Check sheet for the modelled part. Datum: model origin and axes. Units: mm. Face numbers are marked on the shaded views. A direction names the side the tool comes from. Give positions to 0.01 mm unless a question says otherwise; leave off trailing zeros. Write each loop counter-clockwise with the first axis right and the second up, starting at its lowest first coordinate (ties: lowest second). Pieces come first, ordered by that corner, then holes. Notation, with made-up numbers: M 1.5,25 L 16.5,25 A13 ccw 16.5,32 Z; hole C -27,85 d1. An arc over 180 degrees is marked long. Write each question's results on one line, items separated by ' | '. Start each with the question number.
from build123d import *

# Parameters (mm, degrees)
SKETCH1_W           = 10
SKETCH1_H           = 10
BOSS_EXTRUDE1_DEPTH = 50
SKETCH3_W           = 10
SKETCH3_H           = 10
BOSS_EXTRUDE3_DEPTH = 11
SKETCH8_W           = 20
SKETCH8_H           = 10
BOSS_EXTRUDE4_DEPTH = 23
SKETCH9_R           = 2
CUT_EXTRUDE2_DEPTH  = 23
SKETCH9_4_R         = 2
CUT_EXTRUDE3_DEPTH  = 23
SKETCH8_4_W         = 20
SKETCH8_4_H         = 10
BOSS_EXTRUDE5_DEPTH = 31
SKETCH8_5_W         = 20
SKETCH8_5_H         = 10
BOSS_EXTRUDE6_DEPTH = 31.5


with BuildPart() as part:
    # Sketch1 → Boss-Extrude1 (new body)
    with BuildSketch(Plane.XY):
        with Locations((-2.851282988, -1.356707317)):
            Rectangle(SKETCH1_W, SKETCH1_H)
    extrude(amount=BOSS_EXTRUDE1_DEPTH)

    # Sketch3 → Boss-Extrude3 (add)
    with BuildSketch(Plane.ZY.offset(7.851282988)):
        with Locations((45, -1.356707317)):
            Rectangle(SKETCH3_W, SKETCH3_H)
    extrude(amount=BOSS_EXTRUDE3_DEPTH)

    # Sketch8 → Boss-Extrude4 (add)
    with BuildSketch(Plane(origin=(0, 3.643292683, 0), x_dir=(1, 0, 0), z_dir=(0, 1, 0))):
        with Locations((-8.851282988, -45)):
            Rectangle(SKETCH8_W, SKETCH8_H)
    extrude(amount=BOSS_EXTRUDE4_DEPTH)

    # Sketch9 → Cut-Extrude2 (cut)
    with BuildSketch(Plane(origin=(0, 3.643292683, 0), x_dir=(1, 0, 0), z_dir=(0, 1, 0))):
        with Locations(Location((-2.851282988, -7, 0), (0, 0, 270))):
            Circle(SKETCH9_R)
    extrude(amount=-CUT_EXTRUDE2_DEPTH, mode=Mode.SUBTRACT)

    # Sketch9<4> → Cut-Extrude3 (cut)
    with BuildSketch(Plane(origin=(0, 3.643292683, 0), x_dir=(1, 0, 0), z_dir=(0, 1, 0))):
        with Locations(Location((-2.851282988, -26, 0), (0, 0, 270))):
            Circle(SKETCH9_4_R)
    extrude(amount=-CUT_EXTRUDE3_DEPTH, mode=Mode.SUBTRACT)

    # Sketch8<4> → Boss-Extrude5 (add)
    with BuildSketch(Plane(origin=(0, 3.643292683, 0), x_dir=(1, 0, 0), z_dir=(0, 1, 0))):
        with Locations((-8.851282988, -45)):
            Rectangle(SKETCH8_4_W, SKETCH8_4_H)
    extrude(amount=BOSS_EXTRUDE5_DEPTH)

    # Sketch8<5> → Boss-Extrude6 (add)
    with BuildSketch(Plane(origin=(0, 3.643292683, 0), x_dir=(1, 0, 0), z_dir=(0, 1, 0))):
        with Locations((-8.851282988, -45)):
            Rectangle(SKETCH8_5_W, SKETCH8_5_H)
    extrude(amount=BOSS_EXTRUDE6_DEPTH)


solid = part.part
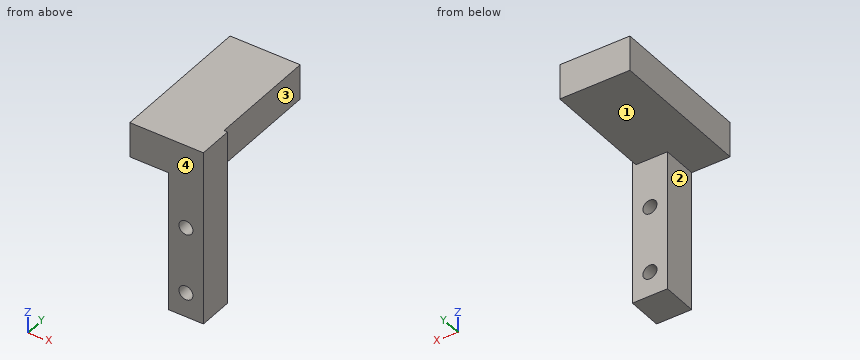
Q1. Tool access check on the marked faces 1, 2, 3 and 4. Record the directions out of +Z, -Z, +X, -X, +Y, -Y that give a thin tool (end or side, any length) a straight path to the whole face; none if there is none.
Q2. Section check B-B on x = -7. Record the boundary of the cut face in (y, z).
Q3. Section check C-C on z = 46. Record the boundary of the cut face in (x, y), plus the area to 3 significant figures.
Q4. Scan lines: L1, parallel to Z at x = -4, y = -4; L2, parallel to X at y = 0.25, z = 7; L3, parallel to Y at x = -4, z = 39.5. Record each from-to range of solid material in increasing order.
Q5. Section check A-A on z = 7. Record the boundary of the cut face in (x, y).
Q6. Section check D-D on y = 29.5. Record the boundary of the cut face in (x, z), plus the area to 3 significant figures.
Q7. Depth check by flat-ended pin: pin 1 Ø6.5 at (x, z) = (-2.85, 7) entering from -Y; pin 2 Ø6.5 at (x, z) = (-2.85, 26) entering from +Y; pin 3 Ø5 at (y, z) = (-1.5, 14) entering from -X; pin 4 Ø5 at (y, z) = (13, 42.5) entering from +X. Enter the tip coordinate at first touch or a pass-through.
Check result:
1) face 1: -Z, -X, +Y | face 2: -Z, -X, +Y, -Y | face 3: +Z, -Z, +X, +Y | face 4: +Z, -Z, +X, -X, -Y
2) outline: M -6.36,0 L 3.64,0 L 3.64,40 L 35.14,40 L 35.14,50 L -6.36,50 Z
3) outline: M -18.85,-6.36 L 2.15,-6.36 L 2.15,3.64 L 1.15,3.64 L 1.15,35.14 L -18.85,35.14 Z | area: 840 mm^2
4) L1: 0 to 5.36, 8.64 to 24.36, 27.64 to 50 | L2: -7.85 to -4.85, -0.85 to 2.15 | L3: -6.36 to 3.64
5) outline: M -7.85,-6.36 L -4.85,-6.36 L -4.85,3.64 L -7.85,3.64 Z; M -0.85,-6.36 L 2.15,-6.36 L 2.15,3.64 L -0.85,3.64 Z
6) outline: M -18.85,40 L 1.15,40 L 1.15,50 L -18.85,50 Z | area: 200 mm^2
7) pin 1: y = -6.36 | pin 2: y = 3.64 | pin 3: x = -7.85 | pin 4: x = 1.15
